Autodesk Inventor part; units mm, degrees
ref_plane "Work Plane2" through (11.2, 0, 0) normal (1, 0, 0) x (0, 1, 0)
ref_plane "Work Plane4" through (11.1, 0, 0) normal (1, 0, 0) x (0, 0, -1)
ref_plane "XZ Plane" through (0, 0, 0) normal (0, 1, 0) x (-1, 0, 0)
sketch "Sketch1" plane through (0, 0, 0) normal (0, 0, 1) x (1, 0, 0)
  line L0 (0, 0) -> (22.2, 0)
  line L1 (22.2, 0) -> (22.2, 22.2)
  line L2 (22.2, 22.2) -> (0, 22.2)
  line L3 (0, 22.2) -> (0, 0)
  dimension "d0" = 22.2
  dimension "d1" = 22.2
extrude "Extrusion1" add sketch "Sketch1" along normal blind 8
sketch "Sketch2" plane through (0, 0, 8) normal (0, 0, 1) x (1, 0, 0)
  line L0 (0, 0) -> (22.2, 0) construction
  line L1 (22.2, 0) -> (22.2, 22.2) construction
  line L2 (22.2, 22.2) -> (0, 22.2) construction
  line L3 (0, 22.2) -> (0, 0) construction
  line L4 (22.2, 22.2) -> (0, 22.2) construction
  line L5 (11.1, 22.2) -> (11.1, 0) construction
  line L6 (0, 0) -> (22.2, 0) construction
  circle A0 centre (11.1, 11.1) radius 8
  dimension "d4" = 16
extrude "Extrusion2" add sketch "Sketch2" along normal blind 7.25
sketch "Sketch3" plane through (22.2, 0, 0) normal (1, 0, 0) x (0, 0, -1)
  line L0 (-15.25, 19.1) -> (-15.25, 3.1) construction
  line L1 (-15.25, 11.1) -> (0, 11.1) construction
  line L2 (0, 22.2) -> (0, 0) construction
sketch "Sketch5" plane through (0, 0, 0) normal (0, -1, 0) x (1, 0, 0)
  line L0 (0, 0) -> (22.2, 0) construction
  line L1 (22.2, 0) -> (22.2, 8) construction
  line L2 (0, 8) -> (22.2, 8) construction
  line L3 (0, 0) -> (0, 8) construction
  line L4 (0, 8) -> (22.2, 8) construction
  line L5 (11.1, 8) -> (11.1, 13.5) construction
  arc A0 (22.2, 8) -> (0, 8) centre (11.1, -0.4509) ccw
  line L6 (0, 8) -> (22.2, 8)
  dimension "d9" = 5.5
extrude "Extrusion4" add sketch "Sketch5" against normal up to surface (22.2 mm away)
sketch "Sketch6" plane through (22.2, 0, 0) normal (1, 0, 0) x (0, 0, -1)
  line L0 (0, 0) -> (0, 22.2) construction
  line L1 (0, 22.2) -> (-8, 22.2) construction
  line L2 (-8, 0) -> (-8, 22.2) construction
  line L3 (0, 0) -> (-8, 0) construction
  line L4 (-8, 0) -> (-8, 22.2) construction
  line L5 (-8, 11.1) -> (-13.5, 11.1) construction
  line L6 (0, 22.2) -> (-8, 22.2)
  line L7 (0, 0) -> (-8, 0)
  arc A0 (-8, 22.2) -> (-8, 0) centre (0.4509, 11.1) ccw
  line L8 (-8, 22.2) -> (-8, 0)
  dimension "d12" = 5.5
extrude "Extrusion5" add sketch "Sketch6" against normal up to surface (22.2 mm away)
sketch "Sketch7" plane through (22.2, 0, 0) normal (1, 0, 0) x (0, 0, -1)
  line L0 (0, 0) -> (0, 22.2) construction
  line L1 (0, 22.2) -> (-8, 22.2) construction
  arc A0 (-8, 22.2) -> (-8, 0) centre (0.4509, 11.1) ccw construction
  line L2 (0, 0) -> (-8, 0) construction
  arc A1 (-8, 22.2) -> (-8, 0) centre (0.4509, 11.1) ccw construction
  line L3 (-13.5, 11.1) -> (0, 11.1) construction
  line L4 (0, 22.2) -> (0, 0) construction
  line L5 (-13.5, 11.1) -> (-13.5, 20.6) construction
  line L6 (-13.5, 11.1) -> (-13.5, 1.6) construction
  line L7 (0, 0) -> (-8, 0)
  line L8 (-13.5, 1.6) -> (-8, 0)
  line L9 (-8, 0) -> (-13.5, 0)
  line L10 (0, 0) -> (-8, 0)
  line L11 (-13.5, 0) -> (-13.5, 1.6)
  line L12 (0, 22.2) -> (-8, 22.2)
  line L13 (-13.5, 20.6) -> (-8, 22.2)
  line L14 (-8, 22.2) -> (-13.5, 22.2)
  line L15 (-13.5, 22.2) -> (-13.5, 20.6)
  dimension "d15" = 9.5
extrude "Extrusion6" cut sketch "Sketch7" against normal up to surface (22.2 mm away)
sketch "Sketch9" plane through (0, 0, 15.25) normal (0, 0, 1) x (1, 0, 0)
  arc A0 (17.7247, 6.5709) -> (17.7247, 15.8291) centre (11.2, 11.2) ccw
  arc A1 (17.7247, 15.8291) -> (16.9166, 16.7965) centre (11.2, 11.2) ccw
  arc A2 (16.9166, 16.7965) -> (16.7965, 16.9166) centre (11.2, 11.2) ccw
  arc A3 (16.7965, 16.9166) -> (15.8291, 17.7247) centre (11.2, 11.2) ccw
  arc A4 (15.8291, 17.7247) -> (6.5709, 17.7247) centre (11.2, 11.2) ccw
  arc A5 (6.5709, 17.7247) -> (5.6035, 16.9166) centre (11.2, 11.2) ccw
  arc A6 (5.6035, 16.9166) -> (5.4834, 16.7965) centre (11.2, 11.2) ccw
  arc A7 (5.4834, 16.7965) -> (4.6753, 15.8291) centre (11.2, 11.2) ccw
  arc A8 (4.6753, 15.8291) -> (4.6753, 6.5709) centre (11.2, 11.2) ccw
  arc A9 (4.6753, 6.5709) -> (5.4834, 5.6035) centre (11.2, 11.2) ccw
  arc A10 (5.4834, 5.6035) -> (5.6035, 5.4834) centre (11.2, 11.2) ccw
  arc A11 (5.6035, 5.4834) -> (6.5709, 4.6753) centre (11.2, 11.2) ccw
  arc A12 (6.5709, 4.6753) -> (15.8291, 4.6753) centre (11.2, 11.2) ccw
  arc A13 (15.8291, 4.6753) -> (16.7965, 5.4834) centre (11.2, 11.2) ccw
  arc A14 (16.7965, 5.4834) -> (16.9166, 5.6035) centre (11.2, 11.2) ccw
  arc A15 (16.9166, 5.6035) -> (17.7247, 6.5709) centre (11.2, 11.2) ccw
  circle A16 centre (11.2, 11.2) radius 7.1389
  point P0 (0, 0)
extrude "Extrusion8" add sketch "Sketch9" along normal blind 2.25 contours A16
sketch "Sketch10" plane through (11.2, 11.2, 17.5) normal (0, 0, 1) x (1, 0, 0)
  circle A0 centre (0, 0) radius 8
  circle A1 centre (0, 0) radius 6
  circle A2 centre (0, 0) radius 7
  point P0 (-11.2, -11.2)
  dimension "d25" = 2
  dimension "d36" = 1
extrude "Extrusion9" add sketch "Sketch10" along normal blind 6 contours A1
sketch "Sketch11" plane through (11.2, 11.2, 23.5) normal (0, 0, 1) x (1, 0, 0)
  circle A0 centre (0, 0) radius 6
  circle A1 centre (0, 0) radius 9.28
  point P0 (-11.2, -11.2)
  dimension "d28" = 18.56
extrude "Extrusion10" add sketch "Sketch11" along normal blind 3.5 contours A0 | A1
sketch "Sketch12" plane through (22.2, 0, 0) normal (1, 0, 0) x (0, 0, -1)
  line L0 (-27, 20.48) -> (-27, 1.92) construction
  line L1 (-27, 11.2) -> (0, 11.1) construction
  line L2 (0, 0) -> (0, 22.2) construction
  dimension "d31" = 27.0002
ref_plane "Work Plane2" through (11.2, 0, 0) normal (1, 0, 0) x (0, 1, 0)
sketch "Sketch17" plane through (0, 0, 0) normal (-1, 0, 0) x (0, 0, 1)
  line L0 (0, 22.2) -> (0, 0) construction
  line L1 (0, 0) -> (8, 0) construction
  arc A0 (8, 0) -> (8, 22.2) centre (-0.4509, 11.1) ccw construction
  line L2 (0, 22.2) -> (8, 22.2) construction
  line L3 (0, 22.2) -> (0, 0) construction
  line L4 (0, 11.1) -> (9, 11.1) construction
  line L5 (9, 11.1) -> (9, 8.35) construction
  line L6 (17.5, 17.2) -> (23.5, 17.2) construction
  line L7 (9, 11.1) -> (9, 13.85) construction
  circle A1 centre (9, 8.35) radius 1
  circle A2 centre (9, 13.85) radius 1
  dimension "d48" = 9
  dimension "d49" = 2.75
  dimension "d50" = 2
  dimension "d52" = 2.75
  dimension "d53" = 2
extrude "Extrusion12" cut sketch "Sketch17" against normal through all
ref_plane "Work Plane4" through (11.1, 0, 0) normal (1, 0, 0) x (0, 0, -1)
sketch "Sketch18" plane through (11.1, 0, 0) normal (1, 0, 0) x (0, 0, -1)
  line L0 (0, 0) -> (0, 22.2)
  line L1 (0, 11.1) -> (-43.4569, 11.1)
properties part number "mini predator dummy camera"
Can you work these out from the model? Positions are in its coordinate system, mm. A direction names the side the tool comes from. Coordinates: 2 decimals unless noted, no trailing zeros. Write each loop counter-clockwise with the first axis right and the second up, starting at its lowest first coordinate (ties: lowest second). Pieces come first, ordered by that corner, then holes. Notation, with made-up numbers: (64, 89) -> (88, 89) arc R17 ccw to (88, 103) -> close; hole circle Ø11 at (15, 41.5). An arc over 180 degrees is marked (long way). Write item = value, one per line.
(1) Imagine slicing it at A-A (x = 4.75). Please give me the cut outline in (y, z).
Verdict:
outline = (0, 0) -> (22.2, 0) -> (22.2, 8) -> (21.04, 11.97) -> (17.45, 11.97) arc R13.95 ccw to (15.97, 12.62) -> (15.97, 15.25) -> (14.26, 15.25) -> (14.26, 17.5) -> (8.14, 17.5) -> (8.14, 15.25) -> (6.23, 15.25) -> (6.23, 12.62) arc R13.95 ccw to (4.75, 11.97) -> (1.16, 11.97) -> (0, 8) -> close; (4.53, 23.5) -> (17.87, 23.5) -> (17.87, 27) -> (4.53, 27) -> close; hole circle Ø2 at (8.35, 9); hole circle Ø2 at (13.85, 9)
(2) Imagine slicing it at D-D (x = 14.5). Please give me the cut outline in (y, z), and give its area (3 significant figures).
Verdict:
outline = (0, 0) -> (22.2, 0) -> (22.2, 8) -> (20.72, 13.08) -> (18.34, 13.08) -> (18.34, 15.25) -> (17.53, 15.25) -> (17.53, 17.5) -> (16.21, 17.5) -> (16.21, 23.5) -> (19.87, 23.5) -> (19.87, 27) -> (2.53, 27) -> (2.53, 23.5) -> (6.19, 23.5) -> (6.19, 17.5) -> (4.87, 17.5) -> (4.87, 15.25) -> (3.86, 15.25) -> (3.86, 13.08) -> (1.48, 13.08) -> (0, 8) -> close; hole circle Ø2 at (8.35, 9); hole circle Ø2 at (13.85, 9)
area = 457 mm^2
(3) Imagine slicing it at C-C (z = 9.5). Please give me the cut outline in (x, y), and give its area (3 significant figures).
Verdict:
outline = (0, 1.32) -> (1.32, 1.32) -> (1.32, 0.44) -> (20.88, 0.44) -> (20.88, 1.32) -> (22.2, 1.32) -> (22.2, 7.48) -> (0, 7.48) -> close; (0, 9.22) -> (22.2, 9.22) -> (22.2, 12.98) -> (0, 12.98) -> close; (0, 14.72) -> (22.2, 14.72) -> (22.2, 20.88) -> (20.88, 20.88) -> (20.88, 21.76) -> (1.32, 21.76) -> (1.32, 20.88) -> (0, 20.88) -> close
area = 392 mm^2
(4) On a 3-axis mill with a long thin cutter (end or side, diameter ignored), from which of +Z, -Z, +X, -X, +Y, -Y can I reach the whole of each face in a straight line? I mean faces 1 (the face through (2.2, 11.3, 13.5)), 2 (the face through (3.8, 16.8, 25.2)), 3 (the face through (7, 16, 17.5)), 4 (the face through (11.3, 19.4, 13.5)). Say none if no direction works.
Verdict:
face_1 = -X
face_2 = +Z
face_3 = none
face_4 = +Y
(5) Thinking about a two-plate mould opening in Y: for faces 5 (the face through (10.945, 12.874, 8.783)), 6 (the face through (20.1, 11.3, 13.5)), 7 (the face through (11, 0, 4)), 8 (the face through (10.94, 7.74, 8.21)), which applies, +Y half, -Y half, draft (parallel to the pull), parting line (faces both ways), or undercut?
Verdict:
face_5 = undercut
face_6 = parting line
face_7 = -Y half
face_8 = undercut
(6) For pin 1 (1 mm diameter, centred on y = 4.5, z = 14, fed in from +X); pin 2 (10 mm diameter, centred on x = 20, z = 5, fed in from -Y); pin 3 (12 mm diameter, centred on x = 2.5, z = 24, fed in from +Y); pin 4 (1.2 mm diameter, centred on y = 8.35, z = 9, fed in from +X), each with a flat end and sliding along its axis, tell me the tip position at first contact or that it passes through.
Verdict:
pin_1 = 16.28
pin_2 = 0
pin_3 = 20.08
pin_4 = through
(7) Imagine slicing it at B-B (y = 13.85). Please give me the cut outline in (x, z), and give its area (3 significant figures).
Verdict:
outline = (0, 0) -> (22.2, 0) -> (22.2, 8) -> (0, 8) -> close; (0, 10) -> (22.2, 10) -> (22.2, 13.23) -> (18.61, 13.23) -> (18.61, 15.25) -> (17.83, 15.25) -> (17.83, 17.5) -> (16.58, 17.5) -> (16.58, 23.5) -> (20.09, 23.5) -> (20.09, 27) -> (2.31, 27) -> (2.31, 23.5) -> (5.82, 23.5) -> (5.82, 17.5) -> (4.57, 17.5) -> (4.57, 15.25) -> (3.59, 15.25) -> (3.59, 13.23) -> (0, 13.23) -> close
area = 436 mm^2
(8) If I drill on probe 1 along Z at (x, y) = (6.75, 17.5); probe 2 along Y at (x, z) = (7, 9); probe 3 along Z at (x, y) = (17.75, 9.75), over which ranges is the centre line in solid material (lowest first)?
Verdict:
probe_1 = 0 to 15.25, 23.5 to 27
probe_2 = 0.29 to 7.35, 9.35 to 12.85, 14.85 to 21.91
probe_3 = 0 to 17.5, 23.5 to 27
